Source: CAD feature listing. Evaluate the final solid. Frame: model axes, mm. Face numbers are marked on the shaded views. Round coordinates to 2 decimals unless told otherwise and drop trailing zeros. Loops run counter-clockwise (first coordinate to the right, second up) from the corner with the lowest first, then second, coordinate; pieces in that order, holes last. Notation, with made-up numbers: M 7.5,-19.75 L 16.5,-19.75 A22 ccw 16.5,-2.75 Z; hole C 80.5,63 d2. An arc over 180 degrees is marked long. Write each question's results on one line, items separated by ' | '. Start each with the question number.
1. Ray query, line 1 (Z direction, x = -251, y = -11.5); line 2 (Y direction, x = -245, z = -22.6); line 3 (Y direction, x = -288, z = -34.5). Return the intervals inside material, ascending.
2. Contact query for flat-ended pins moving along their axis: pin 1 Ø4 at (x, y) = (-311, 0) entering from +Z; pin 2 Ø5 at (x, y) = (-269.5, -4.5) entering from +Z; pin 3 Ø10 at (x, z) = (-261.5, -45) entering from +Y. Output: stop coordinate, or through.
3. Section A-A on x = -318. Output: boundary loops of the cut face in (y, z).
4. Draft query along Y for the marked faces 1, 2 and 3. Return one class per face: released by +Y, released by -Y, zero draft, split by the parting line, or undercut.
5. Section B-B on x = -258. Output: boundary loops of the cut face in (y, z).
from build123d import *

# Parameters (mm, degrees)
SKETCH017_R      = 2
EXTRUDE017_DEPTH = 40
SKETCH016_R      = 2.75
EXTRUDE016_DEPTH = 40
SKETCH015_R      = 20
SKETCH015_R_2    = 16.25
EXTRUDE015_DEPTH = 10
FILLET013_R      = 1
FILLET014_R      = 2


with BuildPart() as extrude017:
    # Sketch017 → Extrude017 (new body)
    with BuildSketch(Plane.XY.offset(-60)):
        with Locations((-245, 0)):
            Circle(SKETCH017_R)
    extrude(amount=EXTRUDE017_DEPTH)


with BuildPart() as fusion134:
    # Sketch016 → Extrude016 (new body)
    with BuildSketch(Plane.XZ.offset(-20)):
        with Locations((-245, -40)):
            Circle(SKETCH016_R)
    extrude(amount=EXTRUDE016_DEPTH)

    # Fusion134: union Extrude017
    add(extrude017.part)


with BuildPart() as extrude015:
    # Sketch015 → Extrude015 (new body)
    with BuildSketch(Plane.YZ.offset(-250)):
        with Locations((0, -40)):
            Circle(SKETCH015_R)
        with Locations((0, -40)):
            Circle(SKETCH015_R_2, mode=Mode.SUBTRACT)
    extrude(amount=EXTRUDE015_DEPTH)


with BuildPart() as sphere:
    # Sphere → Sphere (revolve)
    with BuildSketch(Plane(origin=(-318, 0, 0), x_dir=(1, 0, 0), z_dir=(0, -1, 0))):
        with BuildLine():
            ThreePointArc((0, -0.5), (0.5, 0), (0, 0.5))
            Line((0, 0.5), (0, -0.5))
        make_face()
    revolve(axis=Axis((-318, 0, 0), (0, 0, 1)))


with BuildPart() as cone006:
    # Cone006 → Cone006 (revolve)
    with BuildSketch(Plane(origin=(-308, 0, 0), x_dir=(0, 0, -1), z_dir=(0, -1, 0))):
        Polygon((0, 0), (16.25, 82.25), (0, 82.25), align=None)
    revolve(axis=Axis((-308, 0, 0), (1, 0, 0)))


with BuildPart() as obj1:
    # Cone005 → Cone005 (revolve)
    with BuildSketch(Plane(origin=(-308, 0, 0), x_dir=(0, 0, -1), z_dir=(0, -1, 0))):
        Polygon((0, 0), (0.5, 0), (19, 82.25), (0, 82.25), align=None)
    revolve(axis=Axis((-308, 0, 0), (1, 0, 0)))

    # Cut015: cut Cone006
    add(cone006.part, mode=Mode.SUBTRACT)


with BuildPart() as obj1_1:
    # Cut015 placement: moved
    add(obj1.part.moved(Location((-10, 0, 0))))

    # Fusion127: union Sphere
    add(sphere.part)


with BuildPart() as obj1_2:
    # Fusion127 placement: moved
    add(obj1_1.part.moved(Location((-9, 0, -40))))

    # Fusion135: union Extrude015
    add(extrude015.part)

    # Cut019: cut Fusion134
    add(fusion134.part, mode=Mode.SUBTRACT)

    # Fillet013
    fillet013_edges = [obj1_2.edges().sort_by_distance(p)[0] for p in [
        (-250, -20, -40),
        (-240, -20, -40),
        (-250, 0, -22.180851),
    ]]
    fillet(fillet013_edges, radius=FILLET013_R)

    # Fillet014
    fillet014_edges = [obj1_2.edges().sort_by_distance(p)[0] for p in [
        (-240, -16.25, -40),
    ]]
    fillet(fillet014_edges, radius=FILLET014_R)


solid = obj1_2.part
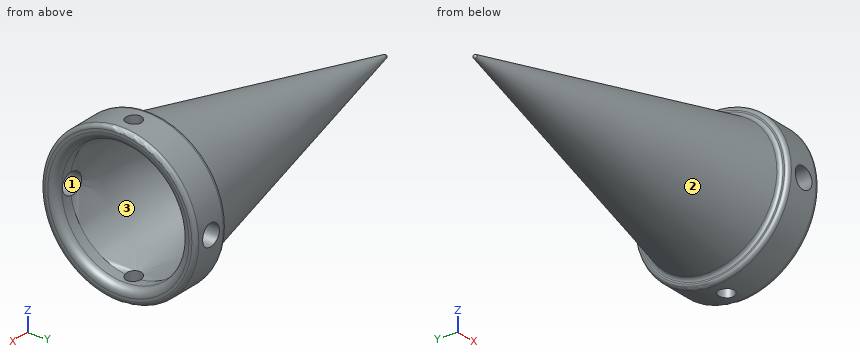
Taken from the geometry:
1) line 1: -53.32 to -49.65, -30.35 to -26.68 | line 2: -9.86 to -2, 2 to 9.86 | line 3: -7.46 to -5.4, 5.4 to 7.46
2) pin 1: z = -35.45 | pin 2: z = -26.44 | pin 3: y = 16.01
3) outline: C 0,-40 d5.05; hole C 0,-40 d3.56
4) face 1: zero draft | face 2: split by the parting line | face 3: undercut
5) outline: C 0,-40 d32.04; hole C 0,-40 d27.26
